from build123d import *

# Parameters (mm, degrees)
SKETCH_2_R      = 82.5
SKETCH_2_R_2    = 1.6
EXTRUDE_1_DEPTH = 3.5
EXTRUDE_2_DEPTH = 8


with BuildPart() as part:
    # Sketch 2 → Extrude 1 (new body)
    with BuildSketch(Plane(origin=(0, 0, 0), x_dir=(1, 0, 0), z_dir=(0, 1, 0))):
        with Locations(Location((0, 0, 0), (0, 0, 270))):
            Circle(SKETCH_2_R)
        with Locations(Location((0, 0, 0), (0, 0, 270))):
            Circle(SKETCH_2_R_2, mode=Mode.SUBTRACT)
        with Locations(Location((0, 7, 0), (0, 0, 270))):
            Circle(SKETCH_2_R_2, mode=Mode.SUBTRACT)
        with Locations(Location((7, 0, 0), (0, 0, 270))):
            Circle(SKETCH_2_R_2, mode=Mode.SUBTRACT)
        with Locations(Location((0, -7, 0), (0, 0, 270))):
            Circle(SKETCH_2_R_2, mode=Mode.SUBTRACT)
        with Locations(Location((-7, 0, 0), (0, 0, 270))):
            Circle(SKETCH_2_R_2, mode=Mode.SUBTRACT)
    extrude(amount=EXTRUDE_1_DEPTH)

    # Sketch 2_3 → Extrude 2 (add)
    with BuildSketch(Plane(origin=(0, 0, 0), x_dir=(1, 0, 0), z_dir=(0, 1, 0))):
        with BuildLine():
            ThreePointArc((57.584494277, -40.978970447), (17.339664943, -23.866001334), (21.17872953, -67.4293068))
            Line((21.17872953, -67.4293068), (19.363549375, -68.748112378))
            ThreePointArc((19.363549375, -68.748112378), (16.164094438, -22.247967345), (59.399674432, -39.660164868))
            Line((59.399674432, -39.660164868), (57.584494277, -40.978970447))
        make_face()
        with BuildLine():
            ThreePointArc((-70.673668965, -0.694632994), (-28.056167231, 9.116001334), (-56.767904218, 42.10291024))
            Line((-56.767904218, 42.10291024), (-56.074567095, 44.236782491))
            ThreePointArc((-56.074567095, 44.236782491), (-26.154054198, 8.497967345), (-71.367006089, -2.828505245))
            Line((-71.367006089, -2.828505245), (-70.673668965, -0.694632994))
        make_face()
        with BuildLine():
            ThreePointArc((-21.17872953, -67.4293068), (-17.339664943, -23.866001334), (-57.584494277, -40.978970447))
            Line((-57.584494277, -40.978970447), (-59.399674432, -39.660164868))
            ThreePointArc((-59.399674432, -39.660164868), (-16.164094438, -22.247967345), (-19.363549375, -68.748112378))
            Line((-19.363549375, -68.748112378), (-21.17872953, -67.4293068))
        make_face()
        with BuildLine():
            ThreePointArc((56.767904218, 42.10291024), (28.056167231, 9.116001334), (70.673668965, -0.694632994))
            Line((70.673668965, -0.694632994), (71.367006089, -2.828505245))
            ThreePointArc((71.367006089, -2.828505245), (26.154054198, 8.497967345), (56.074567095, 44.236782491))
            Line((56.074567095, 44.236782491), (56.767904218, 42.10291024))
        make_face()
        with BuildLine():
            ThreePointArc((-22.5, 67), (0, 29.5), (22.5, 67))
            Line((22.5, 67), (24.743686063, 67))
            ThreePointArc((24.743686063, 67), (0, 27.5), (-24.743686063, 67))
            Line((-24.743686063, 67), (-22.5, 67))
        make_face()
    extrude(amount=EXTRUDE_2_DEPTH)


solid = part.part
Can you work these out from the model? Positions are in its coordinate system, mm. A direction names the side the tool comes from. Round coordinates to 2 decimals unless told otherwise and drop trailing zeros. Loops run counter-clockwise (first coordinate to the right, second up) from the corner with the lowest first, then second, coordinate; pieces in that order, holes last. Notation, with made-up numbers: (-2.75, -33.75) - (12.25, -33.75) arc R21 ccw to (12.25, -8.75) - close; hole circle Ø10 at (12, -26). An arc over 180 degrees is marked (long way). Write item = value, one per line. Start each with the question number.
(1) If we section it at A-A (y = 5.75): Please give me the cut outline in (x, z), and give its area (3 significant figures).
(2) If we section it at C-C (z = -55): Please give me the cut outline in (x, y).
(3) If we section it at B-B (x = 48): Please give me the cut outline in (y, z).
(4) If I drill on probe 1 along Z at (x, y) = (40.5, 4.25); probe 2 along Z at (x, y) = (-40, 6); probe 3 along Y at (x, z) = (25, 34), over which ranges is the centre line in solid material (lowest first)? Write a range as [from, to].
(5) If we mould it in two halves opening along X, with no side actions, what happens to faces 1 (the face through (-17, 0, -1)), 2 (the face through (-0.74, 5.72, -29.51)), 3 (the face through (-80.54, 1.73, -17.88)), 4 (the face through (0.78, 5.72, -27.51))? For each: released by +X, released by -X, zero draft, split by the parting line, or undercut.
(6) For faces 5 (the face through (-16.8, 5.7, 21.8)), 6 (the face through (14, 8, 26)), which set-ups out of +Z, -Z, +X, -X, +Y, -Y let a thin tool reach every point of the face, with its end or its side?
(7) If we section it at D-D (z = 62.5): Please give me the cut outline in (x, y), and give its area (3 significant figures).
(8) For P1, Ø2.5, axis at x = 24, y = 6.5, coming from the -Z side; P2, Ø2, axis at x = 41, z = -57.5, coming from the +Y side; P3, Ø1.9, axis at x = 7, z = 0, coming from the -Y side; P4, Ø1, axis at x = 62, y = 1.5, coming from the +Z side, each with a flat end and sliding along its axis, tell me the tip position at first contact or that it passes through.
Ans:
q1.outline = (-71.37, 2.83) - (-70.67, 0.69) arc R25.5 cw (long way) to (-56.77, -42.1) - (-56.07, -44.24) arc R27.5 ccw (long way) to start; (-59.4, 39.66) arc R27.5 ccw (long way) to (-19.36, 68.75) - (-21.18, 67.43) arc R25.5 cw (long way) to (-57.58, 40.98) - close; (-24.74, -67) - (-22.5, -67) arc R25.5 cw (long way) to (22.5, -67) - (24.74, -67) arc R27.5 ccw (long way) to start; (19.36, 68.75) arc R27.5 ccw (long way) to (59.4, 39.66) - (57.58, 40.98) arc R25.5 cw (long way) to (21.18, 67.43) - close; (56.07, -44.24) - (56.77, -42.1) arc R25.5 cw (long way) to (70.67, 0.69) - (71.37, 2.83) arc R27.5 ccw (long way) to start
q1.area = 1,080 mm²
q2.outline = (-61.49, 0) - (61.49, 0) - (61.49, 3.5) - (27.5, 3.5) - (27.5, 8) - (25.5, 8) - (25.5, 3.5) - (-25.5, 3.5) - (-25.5, 8) - (-27.5, 8) - (-27.5, 3.5) - (-61.49, 3.5) - close
q3.outline = (0, -67.1) - (3.5, -67.1) - (3.5, -44.16) - (8, -44.16) - (8, -42.13) - (3.5, -42.13) - (3.5, 8.14) - (8, 8.14) - (8, 10.16) - (3.5, 10.16) - (3.5, 21.9) - (8, 21.9) - (8, 24.38) - (3.5, 24.38) - (3.5, 67.1) - (0, 67.1) - close
q4.probe_1 = [-41.83, -39.6], [5.61, 7.84], [18.24, 20.34]
q4.probe_2 = [-41.59, -39.33], [5.34, 7.6], [18.09, 20.18]
q4.probe_3 = [0, 3.5]
q5.face_1 = zero draft
q5.face_2 = undercut
q5.face_3 = split by the parting line
q5.face_4 = undercut
q6.face_5 = +Y
q6.face_6 = +Z, -Z, +X, -X, +Y
q7.outline = (-53.85, 0) - (53.85, 0) - (53.85, 3.5) - (14.27, 3.5) - (14.27, 8) - (11.54, 8) - (11.54, 3.5) - (-11.54, 3.5) - (-11.54, 8) - (-14.27, 8) - (-14.27, 3.5) - (-53.85, 3.5) - close
q7.area = 402 mm²
q8.P1 = -67
q8.P2 = 3.5
q8.P3 = through
q8.P4 = 54.99
